Here's how the part is built. I have some questions about the finished solid (model axes, mm). Face numbers are marked on the shaded views. A direction names the side the tool comes from. Coordinates: 2 decimals unless noted, no trailing zeros. Write each loop counter-clockwise with the first axis right and the second up, starting at its lowest first coordinate (ties: lowest second). Pieces come first, ordered by that corner, then holes.
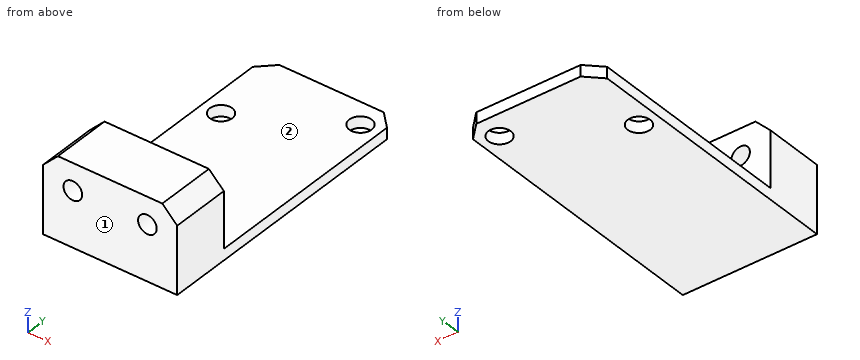
from build123d import *

# Parameters (mm, degrees)
SKETCH1_W             = 18
SKETCH1_H             = 38
EXTRUDE1_DEPTH        = 11
SKETCH2_W             = 18
SKETCH2_H             = 30
EXTRUDE2_DEPTH        = 9.5
SKETCH3_R             = 1.5
EXTRUDE3_DEPTH        = 1.5
SKETCH4_R             = 1.25
EXTRUDE5_DEPTH        = 8
M3_TAPPED_HOLE3_D     = 2.5
M3_TAPPED_HOLE3_DEPTH = 11.5
M3_TAPPED_HOLE3_TIP   = 0.751075774
CHAMFER2_SIZE         = 2


with BuildPart() as part:
    # Sketch1 → Extrude1 (new body)
    with BuildSketch(Plane.XY):
        with Locations((0, -12)):
            Rectangle(SKETCH1_W, SKETCH1_H)
    extrude(amount=EXTRUDE1_DEPTH)

    # Sketch2 → Extrude2 (cut)
    with BuildSketch(Plane.XY.offset(11)):
        with Locations((0, -8)):
            Rectangle(SKETCH2_W, SKETCH2_H)
    extrude(amount=-EXTRUDE2_DEPTH, mode=Mode.SUBTRACT)

    # Sketch3 → Extrude3 (cut)
    with BuildSketch(Plane.XY.offset(1.5)):
        with Locations((6.443229004, 3.72)):
            Circle(SKETCH3_R)
        with Locations((-6.443229004, -3.72)):
            Circle(SKETCH3_R)
    extrude(amount=-EXTRUDE3_DEPTH, mode=Mode.SUBTRACT)

    # Sketch4 → Extrude5 (cut)
    with BuildSketch(Plane(origin=(0, -23, 0), x_dir=(1, 0, 0), z_dir=(0, 1, 0))):
        with Locations(Location((-5, -7.4, 0), (0, 0, 180))):
            Circle(SKETCH4_R)
        with Locations(Location((5, -7.4, 0), (0, 0, 180))):
            Circle(SKETCH4_R)
    extrude(amount=-EXTRUDE5_DEPTH, mode=Mode.SUBTRACT)

    # M3 Tapped Hole3
    with Locations(Plane(origin=(5, -31, 7.4), x_dir=(0, 0, -1), z_dir=(0, -1, 0))):
        with Locations((0, 0), (0, -10)):
            Hole(M3_TAPPED_HOLE3_D / 2, depth=M3_TAPPED_HOLE3_DEPTH)
            with Locations((0, 0, -(M3_TAPPED_HOLE3_DEPTH + M3_TAPPED_HOLE3_TIP / 2))):  # 118° drill point
                Cone(0, M3_TAPPED_HOLE3_D / 2, M3_TAPPED_HOLE3_TIP, mode=Mode.SUBTRACT)

    # Chamfer2
    chamfer2_edges = [part.edges().sort_by_distance(p)[0] for p in [
        (9, -27, 11),
        (-9, -27, 11),
        (-9, 7, 0.75),
        (9, 7, 0.75),
    ]]
    chamfer(chamfer2_edges, length=CHAMFER2_SIZE)


solid = part.part
1. For pin 1 Ø5 at (x, y) = (-6.44, -3.72) entering from +Z; pin 2 Ø2.5 at (x, y) = (6.44, 3.72) entering from -Z; pin 3 Ø3 at (x, z) = (2, 6.5) entering from +Y, each with a flat end and sliding along its axis, tell me the tip position at first contact or that it passes through.
2. I want a section at A-A (z = 7.4). List the corners of the cut face in (x, y) for me, then the cut area to 3 significant figures.
3. On a 3-axis mill with a long thin cutter (end or side, diameter ignored), from which of +Z, -Z, +X, -X, +Y, -Y can I reach the whole of each face in a straight line? I mean the marked faces 1 and 2. Say none if no direction works.
4. I want a section at D-D (x = -1.25). List the corners of the cut face in (y, z) for me.
5. I want a section at B-B (y = -3.72). List the corners of the cut face in (x, z) for me, then the cut area to 3 significant figures.
6. If I drill on line 1 (X direction, y = -28.5, z = 7.4); line 2 (Z direction, x = -5, y = -24.5); line 3 (Z direction, x = 2, y = -16), over which ranges is the centre line in solid material (lowest first)?
7. I want a section at C-C (y = -24.5). List the corners of the cut face in (x, z) for me.
Response values:
1. pin 1: stops at z = 1.5
1. pin 2: passes through
1. pin 3: stops at y = -23
2. outline: (-9, -31) - (-6.25, -31) - (-6.25, -23) - (-9, -23) - close; (-3.75, -31) - (3.75, -31) - (3.75, -23) - (-3.75, -23) - close; (6.25, -31) - (9, -31) - (9, -23) - (6.25, -23) - close
2. area: 104 mm2
3. face 1: +Z, -Z, +X, -X, -Y
3. face 2: +Z, +X, -X, +Y
4. outline: (-31, 0) - (7, 0) - (7, 1.5) - (-23, 1.5) - (-23, 11) - (-31, 11) - close
5. outline: (-9, 0) - (-7.94, 0) - (-7.94, 1.5) - (-9, 1.5) - close; (-4.94, 0) - (9, 0) - (9, 1.5) - (-4.94, 1.5) - close
5. area: 22.5 mm2
6. line 1: x = -9 to -6.25, -3.75 to 3.75, 6.25 to 9
6. line 2: z = 0 to 6.15, 8.65 to 11
6. line 3: z = 0 to 1.5
7. outline: (-9, 0) - (9, 0) - (9, 9) - (7, 11) - (-7, 11) - (-9, 9) - close; hole circle Ø2.5 at (-5, 7.4); hole circle Ø2.5 at (5, 7.4)
